```python
from build123d import *

# Parameters (mm, degrees)
SKETCH1_W           = 40
SKETCH1_H           = 20
BOSS_EXTRUDE1_DEPTH = 40.5
SKETCH2_W           = 20
SKETCH2_H           = 5
BOSS_EXTRUDE2_DEPTH = 7.5
SKETCH3_R           = 2.25
CUT_EXTRUDE1_DEPTH  = 50.964987741
SKETCH4_R           = 4
BOSS_EXTRUDE3_DEPTH = 7.5


with BuildPart() as part:
    # Sketch1 → Boss-Extrude1 (new body)
    with BuildSketch(Plane(origin=(0, 0, 0), x_dir=(1, 0, 0), z_dir=(0, 1, 0))):
        Rectangle(SKETCH1_W, SKETCH1_H)
    extrude(amount=BOSS_EXTRUDE1_DEPTH)

    # Sketch2 → Boss-Extrude2 (add)
    with BuildSketch(Plane(origin=(20, 0, 0), x_dir=(0, 0, -1), z_dir=(1, 0, 0))):
        with Locations((0, 30.05)):
            Rectangle(SKETCH2_W, SKETCH2_H)
    boss_extrude2 = extrude(amount=BOSS_EXTRUDE2_DEPTH)

    # Mirror1: Boss-Extrude2 across plane
    add(boss_extrude2.mirror(Plane(origin=(0, 0, 0), x_dir=(0, 0, 1), z_dir=(1, 0, 0))))

    # Sketch3 → Cut-Extrude1 (cut, through all)
    with BuildSketch(Plane(origin=(0, 0, 0), x_dir=(1, 0, 0), z_dir=(0, 1, 0))):
        with Locations(Location((-24.5, 5, 0), (0, 0, 90))):
            Circle(SKETCH3_R)
        with Locations(Location((24.5, 5, 0), (0, 0, 90))):
            Circle(SKETCH3_R)
        with Locations(Location((24.5, -5, 0), (0, 0, 90))):
            Circle(SKETCH3_R)
        with Locations(Location((-24.5, -5, 0), (0, 0, 90))):
            Circle(SKETCH3_R)
    extrude(amount=CUT_EXTRUDE1_DEPTH, mode=Mode.SUBTRACT)

    # Sketch4 → Boss-Extrude3 (add)
    with BuildSketch(Plane(origin=(0, 40.5, 0), x_dir=(1, 0, 0), z_dir=(0, 1, 0))):
        with Locations(Location((10, 0, 0), (0, 0, 270))):
            Circle(SKETCH4_R)
    extrude(amount=BOSS_EXTRUDE3_DEPTH)


solid = part.part
```
The model under review builds one solid part; all positions refer to its coordinate system, in mm. A direction names the side the tool comes from. Round coordinates to 2 decimals unless told otherwise and drop trailing zeros. Loops run counter-clockwise (first coordinate to the right, second up) from the corner with the lowest first, then second, coordinate; pieces in that order, holes last. Notation, with made-up numbers: (20.25, -34.75) -> (27.25, -34.75) arc R21 ccw to (27.25, -15.75) -> close; hole circle Ø3 at (69.5, 74.25). An arc over 180 degrees is marked (long way). Answer in a Markdown table with one row per item.
1) Wall thickness on line 1 along X through (y, z) = (29.95, -5); line 2 along Z through (x, y) = (-24, 30); line 3 along Y through (x, z) = (-19.5, -7): over which ranges is each line inside the solid? List them lowest first.
Taken from the geometry:
| item | result |
|---|---|
| line 1 | x = -27.5 to -26.75, -22.25 to 22.25, 26.75 to 27.5 |
| line 2 | z = -10 to -7.19, -2.81 to 2.81, 7.19 to 10 |
| line 3 | y = 0 to 40.5 |
2) Tool access review of faces 4 (the flat face through (-20, 14, 0)), 5 (the cylindrical face through (26.696, 30.015, 5.488)), 6 (the flat face through (24, 27.55, 0)), 7 (the flat face through (-20, 36, 0)), 8 (the flat face through (-27.5, 30, 0)): name each direction out of +Z, -Z, +X, -X, +Y, -Y from which nothing blocks a thin tool from reaching the whole face with its end or side.
Taken from the geometry:
| item | result |
|---|---|
| face 4 | +Z, -Z, -X, -Y |
| face 5 | +Y, -Y |
| face 6 | +Z, -Z, +X, -Y |
| face 7 | +Z, -Z, -X, +Y |
| face 8 | +Z, -Z, -X, +Y, -Y |
3) Consider section D-D, the plane x = 10. Write out the cut boundary in (y, z).
Taken from the geometry:
| item | result |
|---|---|
| outline | (0, -10) -> (40.5, -10) -> (40.5, -4) -> (48, -4) -> (48, 4) -> (40.5, 4) -> (40.5, 10) -> (0, 10) -> close |
4) Consider section A-A, the plane z = -5. Write out the cut boundary in (x, y).
Taken from the geometry:
| item | result |
|---|---|
| outline | (-27.5, 27.55) -> (-26.75, 27.55) -> (-26.75, 32.55) -> (-27.5, 32.55) -> close; (-22.25, 27.55) -> (-20, 27.55) -> (-20, 0) -> (20, 0) -> (20, 27.55) -> (22.25, 27.55) -> (22.25, 32.55) -> (20, 32.55) -> (20, 40.5) -> (-20, 40.5) -> (-20, 32.55) -> (-22.25, 32.55) -> close; (26.75, 27.55) -> (27.5, 27.55) -> (27.5, 32.55) -> (26.75, 32.55) -> close |
5) Consider section C-C, the plane z = 0. Write out the cut boundary in (x, y), plus the area to 4 significant figures.
Taken from the geometry:
| item | result |
|---|---|
| outline | (-27.5, 27.55) -> (-20, 27.55) -> (-20, 0) -> (20, 0) -> (20, 27.55) -> (27.5, 27.55) -> (27.5, 32.55) -> (20, 32.55) -> (20, 40.5) -> (14, 40.5) -> (14, 48) -> (6, 48) -> (6, 40.5) -> (-20, 40.5) -> (-20, 32.55) -> (-27.5, 32.55) -> close |
| area | 1,755 mm² |
6) Draft analysis for pull direction Z (two halves, no side actions). For faces 1 (the flat face through (24, 32.55, 0)), 2 (the cylindrical face through (13.966, 44.198, -0.521)), 3 (the cylindrical face through (26.696, 30.015, -4.512)), state which applies: pulls with the +Z half, pulls with the -Z half, needs draft (parallel to the pull), parting line crosses it, or undercut.
Taken from the geometry:
| item | result |
|---|---|
| face 1 | needs draft |
| face 2 | parting line crosses it |
| face 3 | undercut |
7) For pin 1 Ø6 at (y, z) = (14.5, -1) entering from +X; pin 2 Ø4 at (x, z) = (-24.5, 0) entering from +Y; pin 3 Ø6 at (x, z) = (23.5, -1.5) entering from -Y; pin 4 Ø8 at (x, z) = (13, 1) entering from -Y, all flat-tipped, find the tip position at first contact; note any pin that passes through.
Taken from the geometry:
| item | result |
|---|---|
| pin 1 | stops at x = 20 |
| pin 2 | stops at y = 32.55 |
| pin 3 | stops at y = 27.55 |
| pin 4 | stops at y = 0 |
8) Consider section B-B, the plane x = 24.5. Write out the cut boundary in (y, z), plus the area to 3 significant figures.
Taken from the geometry:
| item | result |
|---|---|
| outline | (27.55, -10) -> (32.55, -10) -> (32.55, -7.25) -> (27.55, -7.25) -> close; (27.55, -2.75) -> (32.55, -2.75) -> (32.55, 2.75) -> (27.55, 2.75) -> close; (27.55, 7.25) -> (32.55, 7.25) -> (32.55, 10) -> (27.55, 10) -> close |
| area | 55.0 mm² |
